from build123d import *

# Parameters (mm, degrees)
TAP_DRILL_FOR_M4X0_7_TAP1_D     = 3.3
TAP_DRILL_FOR_M4X0_7_TAP1_DEPTH = 8
TAP_DRILL_FOR_M4X0_7_TAP1_TIP   = 0.991420021
CHAMFER1_SIZE                   = 1
CUT_EXTRUDE3_DEPTH              = 52.479971834
CIRPATTERN2_COUNT               = 4
SKETCH9_R                       = 22.15
SKETCH9_R_2                     = 11.45
CUT_EXTRUDE5_DEPTH              = 2


with BuildPart() as part:
    # Sketch2 → Revolve1 (revolve)
    with BuildSketch(Plane.XY, mode=Mode.PRIVATE) as revolve1_sk:
        Polygon((4, -44.15), (4, 0), (21.692650032, 0), (24.75, -8.4), (14, -8.4), (14, -9.15), (17.75, -9.15), (17.75, -44.15), align=None)
    revolve(revolve1_sk.sketch.rotate(Axis((0, 46.5537, 0), (0, -1, 0)), 90), axis=Axis((0, 46.5537, 0), (0, -1, 0)))

    # Tap Drill for M4x0.7 Tap1
    with Locations(Plane(origin=(0, 0, 0), x_dir=(1, 0, 0), z_dir=(0, 1, 0))):
        with Locations((10.606601718, -10.606601718), (-10.606601718, -10.606601718), (-10.606601718, 10.606601718), (10.606601718, 10.606601718)):
            Hole(TAP_DRILL_FOR_M4X0_7_TAP1_D / 2, depth=TAP_DRILL_FOR_M4X0_7_TAP1_DEPTH)
            with Locations((0, 0, -(TAP_DRILL_FOR_M4X0_7_TAP1_DEPTH + TAP_DRILL_FOR_M4X0_7_TAP1_TIP / 2))):  # 118° drill point
                Cone(0, TAP_DRILL_FOR_M4X0_7_TAP1_D / 2, TAP_DRILL_FOR_M4X0_7_TAP1_TIP, mode=Mode.SUBTRACT)

    # Chamfer1
    chamfer1_edges = [part.edges().sort_by_distance(p)[0] for p in [
        (0, 0, -4),
    ]]
    chamfer(chamfer1_edges, length=CHAMFER1_SIZE)

    # Sketch8 → Cut-Extrude3 (cut, through all)
    with BuildSketch(Plane(origin=(0, -6.4, 0), x_dir=(-1, 0, 0), z_dir=(0, -1, 0))):
        with BuildLine():
            ThreePointArc((-9.95, -22.661862236), (0, -24.75), (9.95, -22.661862236))
            add(Edge.make_bspline(
                [(-9.95, -22.661862236), (-8.05, -7.712712588), (8.05, -7.712712588), (9.95, -22.661862236)],
                knots=[0, 0, 0, 0, 1, 1, 1, 1], degree=3))
        make_face()
    cut_extrude3 = extrude(amount=-CUT_EXTRUDE3_DEPTH, mode=Mode.SUBTRACT)

    # CirPattern2: Cut-Extrude3 ×4 about axis
    cirpattern2_axis = Axis((0, 46.5537, 0), (0, -1, 0))
    for i in range(1, CIRPATTERN2_COUNT):
        add(cut_extrude3.rotate(cirpattern2_axis, i * 360 / CIRPATTERN2_COUNT), mode=Mode.SUBTRACT)

    # Sketch9 → Cut-Extrude5 (cut)
    with BuildSketch(Plane(origin=(0, -6.4, 0), x_dir=(1, 0, 0), z_dir=(0, 1, 0))):
        with Locations(Location((0, 0, 0), (0, 0, 270))):
            Circle(SKETCH9_R)
        with Locations(Location((0, 0, 0), (0, 0, 270))):
            Circle(SKETCH9_R_2, mode=Mode.SUBTRACT)
    extrude(amount=-CUT_EXTRUDE5_DEPTH, mode=Mode.SUBTRACT)


solid = part.part
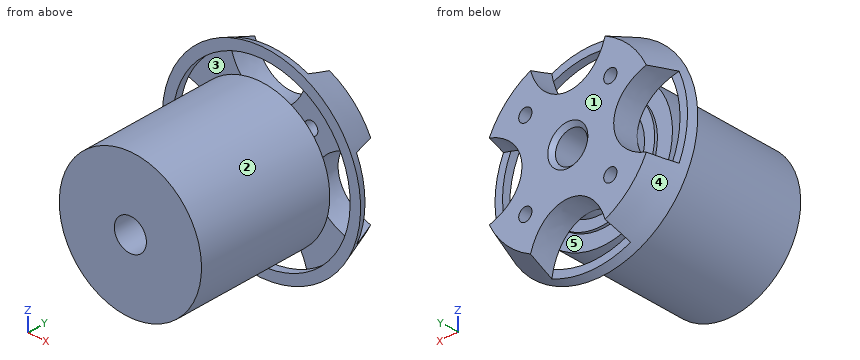
The model under review builds one solid part; all positions refer to its coordinate system, in mm. Face numbers are marked on the shaded views. A direction names the side the tool comes from. Round coordinates to 2 decimals unless told otherwise and drop trailing zeros. Order: outer loops, then holes, each group sorted by start corner. A loop starts at its lowest first (then second) coordinate and runs counter-clockwise, first axis right, second up. Notation, with made-up numbers: (81, 73.25) -> (130, 73.25) arc R17 ccw to (130, 85.25) -> close; hole circle Ø1 at (-27, -7.5). An arc over 180 degrees is marked (long way). Write item = value, one per line. Start each with the question number.
Item 1: Consider section A-A on y = -32. Write out the cut boundary in (x, z), plus the area to 3 significant figures.
Item 2: Mouldability with a two-part tool opening along Y and no side actions: class the marked faces 1, 2 and 3 as released by +Y, released by -Y, zero draft, split by the parting line, or undercut.
Item 3: For line 1 along X through (y, z) = (-13, 0); line 2 along Z through (x, y) = (-7.5, -8); line 3 along X through (y, z) = (-7, 0), list the stretches that pass through material, from the lowest coordinate up.
Item 4: Clearance check with flat-ended pins moving along their axes: pin 1 Ø3 at (x, z) = (4, -22.5) entering from +Y; pin 2 Ø1 at (y, z) = (-38.5, -12.5) entering from -X; pin 3 Ø3 at (y, z) = (-37.5, 6) entering from +X. State where each tip first meets the part, or that it passes through.
Item 5: For the marked faces 4 and 5, list the 3-axis set-ups (+Z, -Z, +X, -X, +Y, -Y) from which the entire face can be reached by the end or side of a thin tool; tool diameter is ignored.
Conclusion:
q1.outline = circle Ø35.5 at (0, 0); hole circle Ø8 at (0, 0)
q1.area = 940 mm2
q2.face_1 = released by +Y
q2.face_2 = zero draft
q2.face_3 = undercut
q3.line_1 = -17.75 to -4, 4 to 17.75
q3.line_2 = -23.43 to -20.84, -8.65 to 8.65, 20.84 to 23.43
q3.line_3 = -24.24 to -22.15, -11.45 to -4, 4 to 11.45, 22.15 to 24.24
q4.pin_1 = -6.4
q4.pin_2 = -13.08
q4.pin_3 = 17.17
q5.face_4 = +Y
q5.face_5 = none
